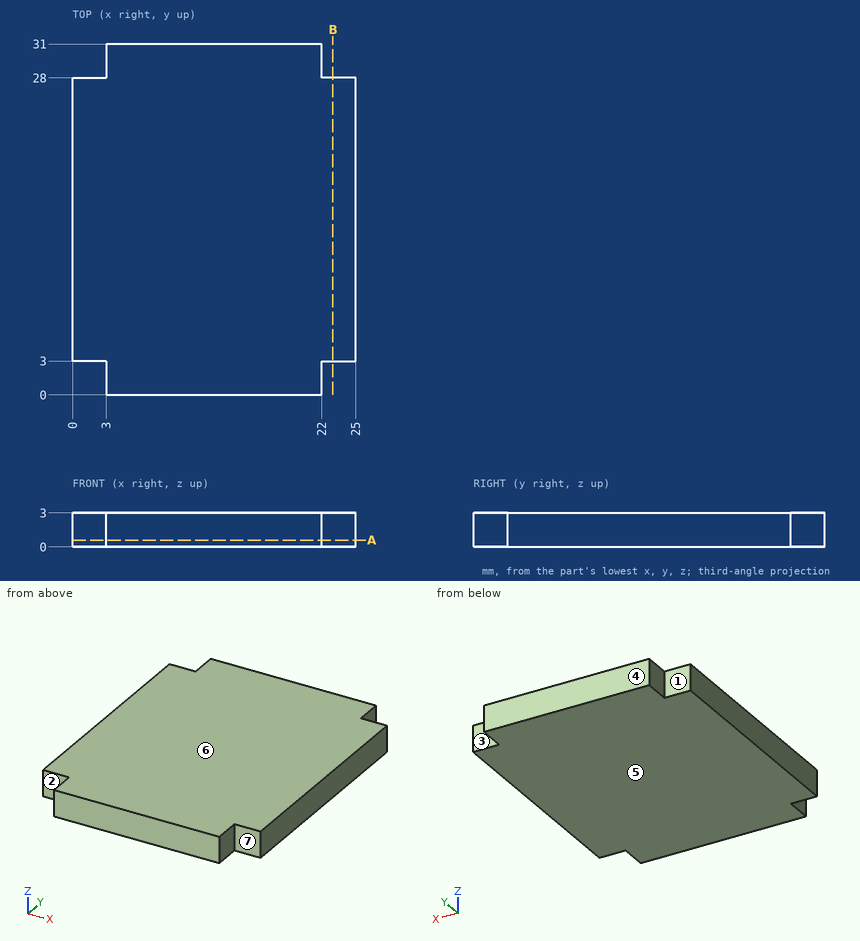
Verification items for this drawing (mm, ordinates from the low corner). A direction names the side the tool comes from. Give positions to 0.01 mm unless a question says otherwise; leave off trailing zeros. Write each loop counter-clockwise with the first axis right and the second up, starting at its lowest first coordinate (ties: lowest second). Pieces come first, ordered by that corner, then holes. Notation, with made-up numbers: (45, 63) -> (66, 63) arc R13 cw to (66, 72) -> close; hole circle Ø3 at (45.5, -12.75). An arc over 180 degrees is marked (long way). Use CSV: the item, a comma, the result in double quotes.
(1) Sectioned sample at A-A (z = 0.6). Record the cut outline in (x, y).
Derived:
outline,"(0, 3) -> (3, 3) -> (3, 0) -> (22, 0) -> (22, 3) -> (25, 3) -> (25, 28) -> (22, 28) -> (22, 31) -> (3, 31) -> (3, 28) -> (0, 28) -> close"
(2) Release check for a two-part mould opening along Z. For the marked faces 5, 6 and 7 record: +Z half, -Z half, draft (parallel to the pull), parting line (faces both ways), or undercut.
Derived:
face 5,"-Z half"
face 6,"+Z half"
face 7,"draft"
(3) Material ranges on L1, parallel to X at y = 29.5, z = 1.6; L2, parallel to Y at x = 23, z = 2.5, recorded low to high.
Derived:
L1,"x = 3 to 22"
L2,"y = 3 to 28"
(4) Go/stop test with flat-tipped pins: pin 1 (1.5 mm diameter, centred on y = 29.5, z = 2, fed in from +X); pin 2 (1 mm diameter, centred on y = 16, z = 1, fed in from -X); pin 3 (0.9 mm diameter, centred on x = 23.5, z = 1.5, fed in from +Y); pin 4 (0.9 mm diameter, centred on x = 1, z = 1, fed in from -Y). Record where each tip stops, or that it passes through.
Derived:
pin 1,"stops at x = 22"
pin 2,"stops at x = 0"
pin 3,"stops at y = 28"
pin 4,"stops at y = 3"
(5) Sectioned sample at B-B (x = 23). Record the cut outline in (y, z).
Derived:
outline,"(3, 0) -> (28, 0) -> (28, 3) -> (3, 3) -> close"
(6) Set-up check for the marked faces 1, 2, 3 and 4: record each of +Z, -Z, +X, -X, +Y, -Y from which the full face is reachable in a straight line by a thin tool's end or side.
Derived:
face 1,"+Z, -Z, -X, +Y"
face 2,"+Z, -Z, -X, -Y"
face 3,"+Z, -Z, +X, +Y"
face 4,"+Z, -Z, +X, -X, +Y"
